Read the model definition and answer for the solid it produces. Units are mm, in the model's axes. Face numbers are marked on the shaded views. A direction names the side the tool comes from. Give positions to 0.01 mm unless a question says otherwise; leave off trailing zeros. Loops run counter-clockwise (first coordinate to the right, second up) from the corner with the lowest first, then second, coordinate; pieces in that order, holes last. Notation, with made-up numbers: (-22, 7) -> (18, 7) arc R7 ccw to (18, 14) -> close; hole circle Ø9 at (-21, 1). An arc over 180 degrees is marked (long way). Return JSON: item names as keys, results as strings. Group by question number.
from build123d import *

# Parameters (mm, degrees)
F0_W     = 50
F0_H     = 26
F1_DEPTH = 77
F2_R     = 5
F4_DEPTH = 25


with BuildPart() as f1:
    # F0 (on Top) → F1 (new body)
    with BuildSketch(Plane.XY):
        Rectangle(F0_W, F0_H)
    extrude(amount=F1_DEPTH)

    # F2
    f2_edges = [f1.edges().sort_by_distance(p)[0] for p in [
        (-25, 0, 0),
        (25, 0, 0),
        (-25, 0, 77),
        (25, 0, 77),
    ]]
    fillet(f2_edges, radius=F2_R)

    # F3 (on face) → F4 (cut)
    with BuildSketch(Plane.XY.offset(77)):
        with BuildLine():
            ThreePointArc((-20, -9.3674969976), (-7.3038475773, -10.8166538264), (-0.5, 0))
            ThreePointArc((-0.5, 0), (-7.3038475773, 10.8166538264), (-20, 9.3674969976))
            Line((-20, 9.3674969976), (-20, -9.3674969976))
        make_face()
        with BuildLine():
            Line((-20, -9.3674969976), (-20, 9.3674969976))
            ThreePointArc((-20, 9.3674969976), (-24.5, 0), (-20, -9.3674969976))
        make_face()
    extrude(amount=-F4_DEPTH, mode=Mode.SUBTRACT)


solid = f1.part
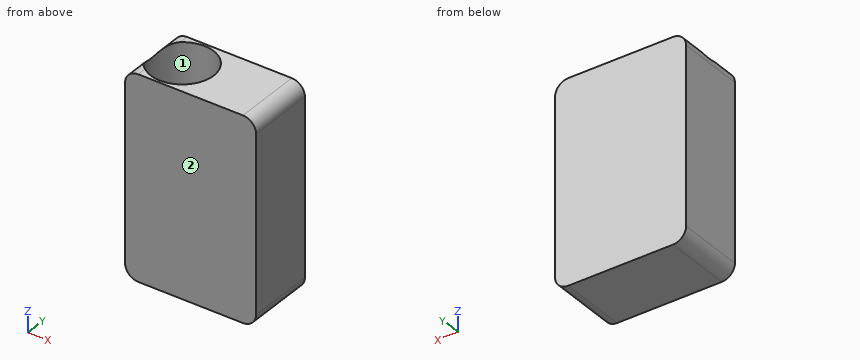
1. Straight lines are drawn through the part: line 1 (Y direction, x = -12, z = 61); line 2 (X direction, y = 0, z = 62); line 3 (Z direction, x = -17, y = 3). For each, find the intervals that lie inside material, in ascending order. Write a range as from..to.
2. Section D-D on y = 7 is taken. Determine the outline of the cut face in (x, z).
3. Section A-A on x = -12.5 is taken. Determine the outline of the cut face in (y, z), then the cut area to 3 significant figures.
4. Section B-B on y = -7.5 is taken. Determine the outline of the cut face in (x, z).
5. Which of the six approach directions +Z, -Z, +X, -X, +Y, -Y give full straight-line access (tool end or side, diameter ignored) to the marked faces 1 and 2?
6. Section C-C on y = -11 is taken. Determine the outline of the cut face in (x, z), then the cut area to 3 significant figures.
Completed:
{
 "1": {"line 1": "y = -13..-11.99, 11.99..13", "line 2": "x = -25..-24.5, -0.5..25", "line 3": "z = 0..52"},
 "2": {"outline": "(-25, 5) arc R5 ccw to (-20, 0) -> (20, 0) arc R5 ccw to (25, 5) -> (25, 72) arc R5 ccw to (20, 77) -> (-2.75, 77) -> (-2.75, 52) -> (-22.25, 52) -> (-22.25, 76.47) arc R5 ccw to (-25, 72) -> close"},
 "3": {"outline": "(-13, 0) -> (13, 0) -> (13, 77) -> (12, 77) -> (12, 52) -> (-12, 52) -> (-12, 77) -> (-13, 77) -> close", "area": "1,400 mm²"},
 "4": {"outline": "(-25, 5) arc R5 ccw to (-20, 0) -> (20, 0) arc R5 ccw to (25, 5) -> (25, 72) arc R5 ccw to (20, 77) -> (-3.13, 77) -> (-3.13, 52) -> (-21.87, 52) -> (-21.87, 76.64) arc R5 ccw to (-25, 72) -> close"},
 "5": {"face 1": "+Z", "face 2": "+Z, -Z, +X, -X, -Y"},
 "6": {"outline": "(-25, 5) arc R5 ccw to (-20, 0) -> (20, 0) arc R5 ccw to (25, 5) -> (25, 72) arc R5 ccw to (20, 77) -> (-7.7, 77) -> (-7.7, 52) -> (-17.3, 52) -> (-17.3, 77) -> (-20, 77) arc R5 ccw to (-25, 72) -> close", "area": "3,590 mm²"}
}
